Check sheet for the modelled part. Datum: model origin and axes. Units: mm. A direction names the side the tool comes from. Round coordinates to 2 decimals unless told otherwise and drop trailing zeros. Loops run counter-clockwise (first coordinate to the right, second up) from the corner with the lowest first, then second, coordinate; pieces in that order, holes last. Notation, with made-up numbers: (85, -2.75) -> (126, -2.75) arc R17 ccw to (126, 15.25) -> close; hole circle Ø8 at (48, 89.5). An arc over 180 degrees is marked (long way). Return JSON: item names as keys, results as strings.
from build123d import *

# Parameters (mm, degrees)
SKETCH1_W           = 3
SKETCH1_H           = 7
BOSS_EXTRUDE1_DEPTH = 157
SKETCH2_W           = 1.5
SKETCH2_H           = 161
BOSS_EXTRUDE2_DEPTH = 3.5
SKETCH3_R           = 1.75
CUT_EXTRUDE1_DEPTH  = 4
CUT_EXTRUDE2_DEPTH  = 4


with BuildPart() as part:
    # Sketch1 → Boss-Extrude1 (new body)
    with BuildSketch(Plane(origin=(0, 0, 0), x_dir=(1, 0, 0), z_dir=(0, 1, 0))):
        with Locations((1.5, 3.5)):
            Rectangle(SKETCH1_W, SKETCH1_H)
    extrude(amount=BOSS_EXTRUDE1_DEPTH)

    # Sketch2 → Boss-Extrude2 (add)
    with BuildSketch(Plane.XY):
        with Locations((2.25, 80.5)):
            Rectangle(SKETCH2_W, SKETCH2_H)
    extrude(amount=BOSS_EXTRUDE2_DEPTH)

    # Sketch3 → Cut-Extrude1 (cut, through all)
    with BuildSketch(Plane(origin=(3, 0, 0), x_dir=(0, 0, -1), z_dir=(1, 0, 0))):
        with Locations((2, 147)):
            Circle(SKETCH3_R)
        with Locations((2, 29)):
            Circle(SKETCH3_R)
    extrude(amount=-CUT_EXTRUDE1_DEPTH, mode=Mode.SUBTRACT)

    # Sketch4 → Cut-Extrude2 (cut, through all)
    with BuildSketch(Plane(origin=(3, 0, 0), x_dir=(0, 0, -1), z_dir=(1, 0, 0))):
        Polygon((-2.485167134, 0), (-3.5, 10.149389846), (-3.5, 0), align=None)
    extrude(amount=-CUT_EXTRUDE2_DEPTH, mode=Mode.SUBTRACT)


solid = part.part
Q1. Go/stop test with flat-tipped pins: pin 1 (1.5 mm diameter, centred on y = 132.5, z = 2, fed in from -X); pin 2 (5.5 mm diameter, centred on y = 147, z = -2, fed in from -X); pin 3 (2 mm diameter, centred on y = 29, z = -2, fed in from -X); pin 4 (0.8 mm diameter, centred on x = 2.5, y = 159, fed in from -Z). Record where each tip stops, or that it passes through.
Results list:
{"pin 1": "x = 1.5", "pin 2": "x = 0", "pin 3": "through", "pin 4": "z = 0"}
Q2. Section check C-C (x = 0.8). Record the boundary of the cut face in (y, z), then the cut area to 3 significant figures.
Results list:
{"outline": "(0, -7) -> (157, -7) -> (157, 0) -> (0, 0) -> close; hole circle Ø3.5 at (29, -2); hole circle Ø3.5 at (147, -2)", "area": "1,080 mm^2"}
Q3. Section check B-B (z = -2). Record the boundary of the cut face in (x, y).
Results list:
{"outline": "(0, 0) -> (3, 0) -> (3, 27.25) -> (0, 27.25) -> close; (0, 30.75) -> (3, 30.75) -> (3, 145.25) -> (0, 145.25) -> close; (0, 148.75) -> (3, 148.75) -> (3, 157) -> (0, 157) -> close"}
Q4. Draft check along Z on faces 1 (the flat face through (1, 77, -7)), 2 (the flat face through (3, 79, -2)), 3 (the cylindrical face through (1.5, 148.5, -2.9)), 4 (the cylindrical face through (1.521, 29.526, -3.669)). Enter one of: released by +Z, released by -Z, zero draft, split by the parting line, or undercut.
Results list:
{"face 1": "released by -Z", "face 2": "zero draft", "face 3": "undercut", "face 4": "undercut"}
Q5. Section check A-A (y = 29). Record the boundary of the cut face in (x, z).
Results list:
{"outline": "(0, -7) -> (3, -7) -> (3, -3.75) -> (0, -3.75) -> close; (0, -0.25) -> (3, -0.25) -> (3, 3.5) -> (1.5, 3.5) -> (1.5, 0) -> (0, 0) -> close"}
Q6. Tool access check on faces 5 (the flat face through (1, 157, -4)), 6 (the flat face through (1.5, 79, 2)), 7 (the flat face through (1, 0, -2)). Record the directions out of +Z, -Z, +X, -X, +Y, -Y that give a thin tool (end or side, any length) a straight path to the whole face; none if there is none.
Results list:
{"face 5": "-Z, +X, -X, +Y", "face 6": "+Z, -X, +Y, -Y", "face 7": "+Z, -Z, +X, -X, -Y"}
Q7. Material ranges on line 1 (Y direction, x = 1, z = -2); line 2 (Z direction, x = 2.2, y = 147); line 3 (Z direction, x = 1.1, y = 147), recorded low to high.
Results list:
{"line 1": "0 to 27.25, 30.75 to 145.25, 148.75 to 157", "line 2": "-7 to -3.75, -0.25 to 3.5", "line 3": "-7 to -3.75, -0.25 to 0"}
